Can you work these out from the drawing? Everything is in mm from the part's minimum corner. Coordinates: 2 decimals unless noted, no trailing zeros. Order: outer loops, then holes, each group sorted by start corner. A loop starts at its lowest first (then second) coordinate and runs counter-clockwise, first axis right, second up. Notation, with made-up numbers: (-2, 43) -> (28, 43) arc R13 ccw to (28, 66) -> close; hole circle Ø3 at (7.5, -14). An arc over 180 degrees is marked (long way). Return JSON: item names as keys, results as strings. Group by question number.
1) If we section it at C-C, the plane z = 10.5: Please give me the cut outline in (x, y), then the cut area to 3 significant figures.
2) If we section it at A-A, the plane y = 2.7: Please give me the cut outline in (x, z), then the cut area to 3 significant figures.
3) If I drill on probe 1 along X at (y, z) = (4.35, 2.5); probe 2 along X at (y, z) = (2.95, 5.5); probe 3 along Z at (x, y) = (16, 1.5), over which ranges is the centre line in solid material (lowest first)? Write a range as from..to.
4) For pin 1 (2 mm diameter, centred on y = 1, z = 11, fed in from -X); pin 2 (1.5 mm diameter, centred on y = 2.5, z = 11, fed in from +X), each with a flat end and sliding along its axis, tell me the tip position at first contact or that it passes through.
5) If we section it at B-B, the plane x = 28.5: Please give me the cut outline in (y, z).
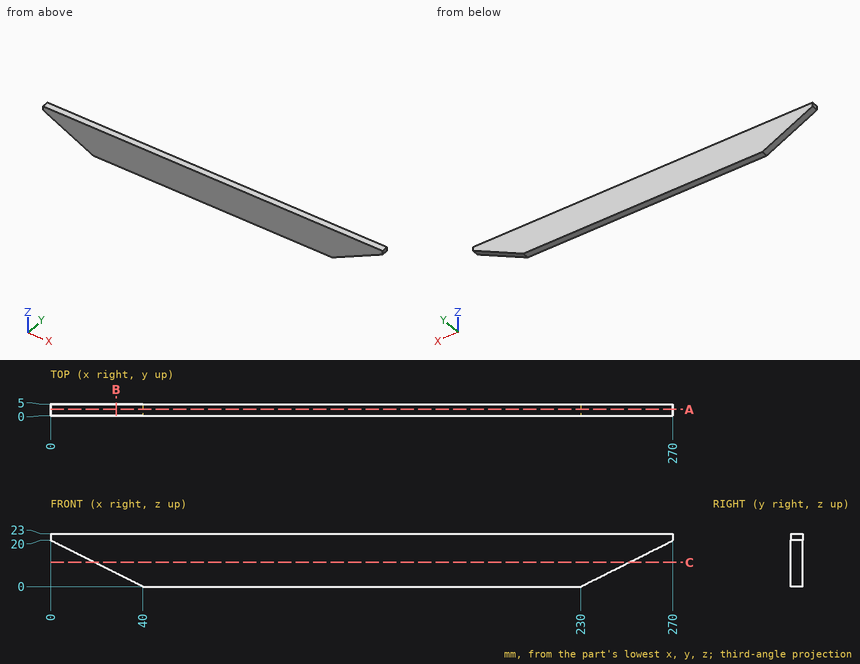
Result sheet:
{
 "1": {"outline": "(19, 0) -> (251, 0) -> (251, 5) -> (19, 5) -> close", "area": "1,160 mm2"},
 "2": {"outline": "(0, 20) -> (40, 0) -> (230, 0) -> (270, 20) -> (270, 23) -> (0, 23) -> close", "area": "5,410 mm2"},
 "3": {"probe 1": "x = 35..235", "probe 2": "x = 29..241", "probe 3": "z = 12..23"},
 "4": {"pin 1": "stops at x = 16", "pin 2": "stops at x = 253.5"},
 "5": {"outline": "(0, 5.75) -> (5, 5.75) -> (5, 23) -> (0, 23) -> close"}
}
